```python
from build123d import *

# Parameters (mm, degrees)
SKIZZE1_W                       = 90
SKIZZE1_H                       = 24
AUFSATZ_LINEAR_AUSTRAGEN1_DEPTH = 62
SKIZZE2_W                       = 86
SKIZZE2_H                       = 58
SCHNITT_LINEAR_AUSTRAGEN1_DEPTH = 22
SKIZZE3_W                       = 58
SKIZZE3_H                       = 20
SCHNITT_LINEAR_AUSTRAGEN2_DEPTH = 5
SKIZZE4_W                       = 67
SKIZZE4_H                       = 16
SCHNITT_LINEAR_AUSTRAGEN3_DEPTH = 50
SKIZZE6_W                       = 3
SKIZZE6_H                       = 80
AUFSATZ_LINEAR_AUSTRAGEN2_DEPTH = 24
SKIZZE5_R                       = 2
SCHNITT_LINEAR_AUSTRAGEN6_DEPTH = 24
VERRUNDUNG1_R                   = 1.5
VERRUNDUNG2_R                   = 1
VERRUNDUNG3_R                   = 0.5


with BuildPart() as part:
    # Skizze1 → Aufsatz-Linear austragen1 (new body)
    with BuildSketch(Plane.XY):
        with Locations((-45, 12)):
            Rectangle(SKIZZE1_W, SKIZZE1_H)
    extrude(amount=-AUFSATZ_LINEAR_AUSTRAGEN1_DEPTH)

    # Skizze2 → Schnitt-Linear austragen1 (cut)
    with BuildSketch(Plane.XZ):
        with Locations((-45, -31)):
            Rectangle(SKIZZE2_W, SKIZZE2_H)
    extrude(amount=-SCHNITT_LINEAR_AUSTRAGEN1_DEPTH, mode=Mode.SUBTRACT)

    # Skizze3 → Schnitt-Linear austragen2 (cut)
    with BuildSketch(Plane.ZY.offset(90)):
        with Locations((-31, 10)):
            Rectangle(SKIZZE3_W, SKIZZE3_H)
    extrude(amount=-SCHNITT_LINEAR_AUSTRAGEN2_DEPTH, mode=Mode.SUBTRACT)

    # Skizze4 → Schnitt-Linear austragen3 (cut)
    with BuildSketch(Plane.XY):
        with Locations((-38.5, 12)):
            Rectangle(SKIZZE4_W, SKIZZE4_H)
    extrude(amount=-SCHNITT_LINEAR_AUSTRAGEN3_DEPTH, mode=Mode.SUBTRACT)

    # Skizze6 → Aufsatz-Linear austragen2 (add)
    with BuildSketch(Plane(origin=(0, 0, 0), x_dir=(1, 0, 0), z_dir=(0, 1, 0))):
        with Locations((1.5, 31)):
            Rectangle(SKIZZE6_W, SKIZZE6_H)
    extrude(amount=AUFSATZ_LINEAR_AUSTRAGEN2_DEPTH)

    # Skizze5 → Schnitt-Linear austragen6 (cut)
    with BuildSketch(Plane(origin=(0, 0, 0), x_dir=(0, 0, -1), z_dir=(1, 0, 0))):
        with Locations(Location((67, 12, 0), (0, 0, 180))):
            Circle(SKIZZE5_R)
        with Locations(Location((-5, 12, 0), (0, 0, 180))):
            Circle(SKIZZE5_R)
    extrude(amount=SCHNITT_LINEAR_AUSTRAGEN6_DEPTH, mode=Mode.SUBTRACT)

    # Verrundung1
    verrundung1_edges = [part.edges().sort_by_distance(p)[0] for p in [
        (0, 12, -62),
        (0, 12, 0),
    ]]
    fillet(verrundung1_edges, radius=VERRUNDUNG1_R)

    # Verrundung2
    verrundung2_edges = [part.edges().sort_by_distance(p)[0] for p in [
        (0, 12, -71),
        (0, 12, 9),
    ]]
    fillet(verrundung2_edges, radius=VERRUNDUNG2_R)

    # Verrundung3
    verrundung3_edges = [part.edges().sort_by_distance(p)[0] for p in [
        (-90, 12, -62),
        (-45.75, 0, -62),
        (0, 0, -66.75),
        (0, 24, -66.75),
        (2, 0, 9),
        (0.292893219, 0, 8.707106781),
        (0.292893219, 0, -70.707106781),
        (2, 24, 9),
        (0.292893219, 24, 8.707106781),
        (0.292893219, 24, -70.707106781),
        (-45.75, 0, 0),
        (-90, 12, 0),
        (2, 0, -71),
        (2, 24, -71),
        (-90, 24, -31),
        (-45.75, 24, 0),
        (0, 0, 4.75),
        (0, 24, 4.75),
        (-45.75, 24, -62),
        (-0.439339828, 24, 0.439339828),
        (-0.439339828, 0, 0.439339828),
        (-0.439339828, 24, -62.439339828),
        (-0.439339828, 0, -62.439339828),
    ]]
    fillet(verrundung3_edges, radius=VERRUNDUNG3_R)


solid = part.part
```
Can you work these out from the model? Positions are in its coordinate system, mm. A direction names the side the tool comes from. Give positions to 0.01 mm unless a question says otherwise; leave off trailing zeros. Loops run counter-clockwise (first coordinate to the right, second up) from the corner with the lowest first, then second, coordinate; pieces in that order, holes last. Notation, with made-up numbers: M 40,-22.5 L 47,-22.5 A15 cw 47,5.5 Z; hole C 10,25 d11. An arc over 180 degrees is marked long. One line per item, written item: value.
(1) Suppose I cut it at A-A on z = -67. List the corners of the cut face in (x, y) for me.
Returned:
outline: M 0,0.5 A0.5 ccw 0.5,0 L 3,0 L 3,10 L 0,10 Z; M 0,14 L 3,14 L 3,24 L 0.5,24 A0.5 ccw 0,23.5 Z
(2) I need wall thicknesses on line 1 (Z direction, x = 0.9, y = 12); line 2 (Y direction, x = 1, z = -67); line 3 (X direction, y = 21.75, z = -3). Which ranges of each line are inside material? Lowest first, please.
Returned:
line 1: -70.99 to -69, -65 to 3, 7 to 8.99
line 2: 0 to 10, 14 to 24
line 3: -90 to -88, -2 to 3
(3) We'd pull the mould along Z, two halves only. Please class faces 1 (the face through (-72, 12, -1)), 2 (the face through (-66, 2, 0)), 3 (the face through (-47, 11, -60)): released by +Z, released by -Z, zero draft, split by the parting line, or undercut.
Returned:
face 1: zero draft
face 2: released by +Z
face 3: undercut
(4) Which directions (+Z, -Z, +X, -X, +Y, -Y) give clear straight access to the entire face, cutting with the end or side of a thin tool? Please do faces 4 (the face through (-88, 21, -31)), 5 (the face through (-5, 12, -1)), 6 (the face through (-46, 12, -62)), 7 (the face through (1.479, 10.648, 3.526)).
Returned:
face 4: -Y
face 5: +Z
face 6: -Z, -X, +Y, -Y
face 7: +X, -X
(5) Suppose I cut it at B-B on y = 12. Count the separate pieces of the cut face and the enclosed holes in it, plus the area to 3 significant figures.
Returned:
separate pieces: 4
enclosed holes: 0
area: 558 mm^2
(6) Suppose I cut it at D-D on x = -3.5. List the corners of the cut face in (y, z) for me, plus the area to 3 significant figures.
Returned:
outline: M 0,-61.5 A0.5 ccw 0.5,-62 L 23.5,-62 A0.5 ccw 24,-61.5 L 24,-0.5 A0.5 ccw 23.5,0 L 0.5,0 A0.5 ccw 0,-0.5 L 0,-2 L 22,-2 L 22,-60 L 0,-60 Z
area: 212 mm^2
(7) Will these pins go through, and if not, where does the flat tip stop? pin 1 (6.5 mm diameter, centred on y = 6, z = -39.5, fed in from -X); pin 2 (12 mm diameter, centred on x = -20.5, y = 7.5, fed in from +Z); pin 3 (1.5 mm diameter, centred on x = -32.5, y = 9.5, fed in from +Z).
Returned:
pin 1: x = -2
pin 2: z = 0
pin 3: z = -60
(8) Suppose I cut it at C-C on x = -63. List the corners of the cut face in (y, z) for me, plus the area to 3 significant figures.
Returned:
outline: M 0,-61.5 A0.5 ccw 0.5,-62 L 23.5,-62 A0.5 ccw 24,-61.5 L 24,-0.5 A0.5 ccw 23.5,0 L 20,0 L 20,-2 L 22,-2 L 22,-60 L 0,-60 Z; M 0,-2 L 4,-2 L 4,0 L 0.5,0 A0.5 ccw 0,-0.5 Z
area: 180 mm^2
